Source: CAD feature listing. Evaluate the final solid. Frame: model axes, mm. A direction names the side the tool comes from. Round coordinates to 2 decimals unless told otherwise and drop trailing zeros. Loops run counter-clockwise (first coordinate to the right, second up) from the corner with the lowest first, then second, coordinate; pieces in that order, holes last.
Item 1: Pull-direction query (X, two-part tool) for faces 3 (the cylindrical face through (-2.539, 19.334, 7.493)), 4 (the cylindrical face through (-28.29, 16.72, 1.97)), 5 (the flat face through (0, 22.5, 2)); classes: released by +X, released by -X, zero draft, split by the parting line, or undercut.
Item 2: Section query A-A on y = 0. Return loops of the section in (x, z), then the cut area to 3 significant figures.
Item 3: Access query for faces 1 (the flat face through (-32.5, 0, 2)), 2 (the flat face through (-22.1, 5.3, 4)). Directions: +Z, -Z, +X, -X, +Y, -Y. A direction counts if a zero-diameter tool reaches every point of the face in a straight line with its end or side. Return the directions, or none.
Item 4: Section query B-B on z = 2.75. Return loops of the section in (x, y), then the cut area to 3 significant figures.
Item 5: First-contact query: P1, Ø1, axis at x = 22, y = -14.5, coming from the -Z side; P2, Ø3, axis at x = 26, y = 16, coming from the +Z side; P3, Ø5, axis at x = -23.5, y = -5.5, coming from the +Z side; P4, Ø4, axis at x = -5.5, z = 7, coming from the +Y side. Flat tips, straight axial feed; report the tip coordinate or a pass-through.
Item 6: Section query C-C on x = 26. Return loops of the section in (y, z), then the cut area to 3 significant figures.
Item 7: Ray query, L1, parallel to Y at x = -26, z = 1.9; L2, parallel to Z at x = -21.5, y = 17; L3, parallel to Y at x = 5, z = 3. Return the intervals inside material, ascending.
```python
from build123d import *

# Parameters (mm, degrees)
SKETCH1_W            = 65
SKETCH1_H            = 45
SKETCH1_R            = 2
BOSS_EXTRUDE1_DEPTH  = 4
SKETCH4_R            = 19.5
SKETCH4_R_2          = 16.5
BOSS_EXTRUDE3_DEPTH  = 4
SKETCH5_R            = 13.5
CUT_EXTRUDE2_DEPTH   = 40.730341051
M4_CLEARANCE_HOLE1_D = 4.8
FILLET1_R            = 3


with BuildPart() as part:
    # Sketch1 → Boss-Extrude1 (new body)
    # profile 1 of 5: a face of its own
    with BuildSketch(Plane.XY):
        Rectangle(SKETCH1_W, SKETCH1_H)
        with Locations((26, 16)):
            Circle(SKETCH1_R, mode=Mode.SUBTRACT)
        with Locations((26, -16)):
            Circle(SKETCH1_R, mode=Mode.SUBTRACT)
        with Locations((-26, -16)):
            Circle(SKETCH1_R, mode=Mode.SUBTRACT)
        with Locations((-26, 16)):
            Circle(SKETCH1_R, mode=Mode.SUBTRACT)
    # profile 2 of 5: a face of its own
    with BuildSketch(Plane.XY):
        with Locations((-26, 16)):
            Circle(SKETCH1_R)
    # profile 3 of 5: a face of its own
    with BuildSketch(Plane.XY):
        with Locations((-26, -16)):
            Circle(SKETCH1_R)
    # profile 4 of 5: a face of its own
    with BuildSketch(Plane.XY):
        with Locations((26, -16)):
            Circle(SKETCH1_R)
    # profile 5 of 5: a face of its own
    with BuildSketch(Plane.XY):
        with Locations((26, 16)):
            Circle(SKETCH1_R)
    extrude(amount=BOSS_EXTRUDE1_DEPTH)

    # Sketch4 → Boss-Extrude3 (add)
    with BuildSketch(Plane.XY.offset(4)):
        Circle(SKETCH4_R)
        Circle(SKETCH4_R_2, mode=Mode.SUBTRACT)
    extrude(amount=BOSS_EXTRUDE3_DEPTH)

    # Sketch5 → Cut-Extrude2 (cut, through all)
    with BuildSketch(Plane.XY.offset(4)):
        Circle(SKETCH5_R)
    extrude(amount=-CUT_EXTRUDE2_DEPTH, mode=Mode.SUBTRACT)

    # M4 Clearance Hole1 (through all)
    with Locations(Plane.XY.offset(4)):
        with Locations((26, 16), (26, -16), (-26, -16), (-26, 16)):
            Hole(M4_CLEARANCE_HOLE1_D / 2)

    # Fillet1
    fillet1_edges = [part.edges().sort_by_distance(p)[0] for p in [
        (-19.5, 0, 4),
        (32.5, -22.5, 2),
        (-32.5, -22.5, 2),
        (-32.5, 22.5, 2),
        (32.5, 22.5, 2),
    ]]
    fillet(fillet1_edges, radius=FILLET1_R - 0.0001)  # a hair under: the kernel refuses the full size


solid = part.part
```
Data:
1. face 3: split by the parting line
1. face 4: undercut
1. face 5: zero draft
2. outline: (-32.5, 0) - (-13.5, 0) - (-13.5, 4) - (-16.5, 4) - (-16.5, 8) - (-19.5, 8) - (-19.5, 7) arc R3 cw to (-22.5, 4) - (-32.5, 4) - close; (13.5, 0) - (32.5, 0) - (32.5, 4) - (22.5, 4) arc R3 cw to (19.5, 7) - (19.5, 8) - (16.5, 8) - (16.5, 4) - (13.5, 4) - close
2. area: 180 mm2
3. face 1: +Z, -Z, -X, +Y, -Y
3. face 2: +Z
4. outline: (-32.5, -19.5) arc R3 ccw to (-29.5, -22.5) - (29.5, -22.5) arc R3 ccw to (32.5, -19.5) - (32.5, 19.5) arc R3 ccw to (29.5, 22.5) - (-29.5, 22.5) arc R3 ccw to (-32.5, 19.5) - close; hole circle Ø4.8 at (-26, -16); hole circle Ø4.8 at (-26, 16); hole circle Ø27 at (0, 0); hole circle Ø4.8 at (26, -16); hole circle Ø4.8 at (26, 16)
4. area: 2,270 mm2
5. P1: stops at z = 0
5. P2: passes through
5. P3: stops at z = 4.13
5. P4: stops at y = 19.58
6. outline: (-22.5, 0) - (-18.4, 0) - (-18.4, 4) - (-22.5, 4) - close; (-13.6, 0) - (13.6, 0) - (13.6, 4) - (-13.6, 4) - close; (18.4, 0) - (22.5, 0) - (22.5, 4) - (18.4, 4) - close
6. area: 142 mm2
7. L1: y = -22.5 to -18.4, -13.6 to 13.6, 18.4 to 22.5
7. L2: z = 0 to 4
7. L3: y = -22.5 to -12.54, 12.54 to 22.5
